The model under review builds one solid part; all positions refer to its coordinate system, in mm. Coordinates: 2 decimals unless noted, no trailing zeros. Write each loop counter-clockwise with the first axis right and the second up, starting at its lowest first coordinate (ties: lowest second). Pieces come first, ordered by that corner, then holes. Notation, with made-up numbers: (24.5, 41.5) - (79.5, 41.5) arc R26 ccw to (79.5, 63.5) - close; hole circle Ø1 at (76, -34.5). An arc over 180 degrees is marked (long way). Put each result on its own line as item: value. Start each with the question number.
Item 1: Consider section B-B on x = 0. Give the boundary of the cut face in (y, z), then the cut area to 3 significant figures.
Item 2: For pin 1 (6.5 mm diameter, centred on x = 2, y = -2, fed in from +Z) (3 decimals); pin 2 (6.5 mm diameter, centred on x = 0.5, y = -2.5, fed in from -Z) (3 decimals); pin 3 (4 mm diameter, centred on y = -6.5, z = -18, fed in from -X); pin 4 (6 mm diameter, centred on x = 2, z = -20.5, fed in from +Y), all flat-tipped, find the tip position at first contact; note any pin that passes through.
Item 3: To check wall thickness, follow L1, parallel to X at y = -5.75, z = 17 (3 decimals); L2, parallel to Z at x = -13, y = -4; L3, parallel to Z at x = -2.5, y = -2.25. State the ranges of each line that lie inside material, in increasing order. Write a range as [from, to].
Item 4: Consider section C-C on y = -3.5. State how many separate pieces and enclosed holes the cut face has, then the cut area to 3 significant figures.
Item 5: Consider section A-A on y = -8.25. Give the boundary of the cut face in (x, z) (1 decimal), then the cut area to 3 significant figures.
```python
from build123d import *

# Parameters (mm, degrees)
F0_R     = 29.845
F1_DEPTH = 6.35
F2_R     = 8.636
F3_DEPTH = 8.89
F4_R     = 1.5875
F5_DEPTH = 15.241
F6_R     = 1.4605
F7_DEPTH = 15.241
F8_R     = 1.4605
F9_DEPTH = 29.846


with BuildPart() as f1:
    # F0 (on Front) → F1 (new body)
    with BuildSketch(Plane.XZ):
        with Locations((0.718291, 0)):
            Circle(F0_R)
        Polygon((-12.740865, -24.658204), (-17.411727, -21.264625), (-16.808232, -15.52275), (-11.533875, -13.174455), (-6.863013, -16.568034), (-7.466508, -22.309909), align=None, mode=Mode.SUBTRACT)
        Polygon((-24.664124, -12.037813), (-26.448234, -6.546885), (-22.585007, -2.256337), (-16.937669, -3.456715), (-15.153559, -8.947643), (-19.016786, -13.238191), align=None, mode=Mode.SUBTRACT)
        Polygon((4.323334, -27.86), (-1.450169, -27.86), (-4.33692, -22.86), (-1.450169, -17.86), (4.323334, -17.86), (7.210085, -22.86), align=None, mode=Mode.SUBTRACT)
        Polygon((20.010529, -20.420223), (15.339667, -23.813802), (10.06531, -21.465507), (9.461815, -15.723632), (14.132676, -12.330053), (19.407034, -14.678348), align=None, mode=Mode.SUBTRACT)
        Polygon((28.328745, -5.180614), (26.544635, -10.671542), (20.897297, -11.87192), (17.034069, -7.581372), (18.81818, -2.090444), (24.465518, -0.890066), align=None, mode=Mode.SUBTRACT)
        Polygon((-26.892163, 5.180614), (-25.108052, 10.671542), (-19.460715, 11.87192), (-15.597487, 7.581372), (-17.381598, 2.090444), (-23.028935, 0.890066), align=None, mode=Mode.SUBTRACT)
        Polygon((-18.573947, 20.420223), (-13.903085, 23.813802), (-8.628728, 21.465507), (-8.025232, 15.723632), (-12.696094, 12.330053), (-17.970451, 14.678348), align=None, mode=Mode.SUBTRACT)
        Polygon((5.773503, 22.86), (2.886751, 17.86), (-2.886751, 17.86), (-5.773503, 22.86), (-2.886751, 27.86), (2.886751, 27.86), align=None, mode=Mode.SUBTRACT)
        Polygon((26.100706, 12.037813), (27.884817, 6.546885), (24.021589, 2.256337), (18.374252, 3.456715), (16.590141, 8.947643), (20.453368, 13.238191), align=None, mode=Mode.SUBTRACT)
        Polygon((14.177448, 24.658204), (18.848309, 21.264625), (18.244814, 15.52275), (12.970457, 13.174455), (8.299595, 16.568034), (8.90309, 22.309909), align=None, mode=Mode.SUBTRACT)
    extrude(amount=F1_DEPTH)

    # F2 (on face) → F3 (join)
    with BuildSketch(Plane.XZ.offset(6.35)):
        with Locations((0.718291, 0)):
            Circle(F2_R)
    extrude(amount=F3_DEPTH)

    # F4 (on face) → F5 (cut, through all)
    with BuildSketch(Plane.XZ.offset(15.24)):
        with Locations((0.718291, 0)):
            Circle(F4_R)
    extrude(amount=-F5_DEPTH, mode=Mode.SUBTRACT)

    # F6 (on face) → F7 (cut, through all)
    with BuildSketch(Plane(origin=(0, 0, 0), x_dir=(-1, 0, 0), z_dir=(0, 1, 0))):
        with Locations((9.9703, 0)):
            Circle(F6_R)
    extrude(amount=-F7_DEPTH, mode=Mode.SUBTRACT)

    # F8 (on Top) → F9 (cut, through all)
    with BuildSketch(Plane.XY):
        with Locations((0, -11.241886)):
            Circle(F8_R)
    extrude(amount=F9_DEPTH, mode=Mode.SUBTRACT)


solid = f1.part
```
Report:
1. outline: (-15.24, -8.61) - (-6.35, -8.61) - (-6.35, -17.86) - (0, -17.86) - (0, -1.42) - (-15.24, -1.42) - close; (-15.24, 1.42) - (-12.7, 1.42) - (-12.7, 8.61) - (-15.24, 8.61) - close; (-9.78, 1.42) - (0, 1.42) - (0, 17.86) - (-6.35, 17.86) - (-6.35, 8.61) - (-9.78, 8.61) - close; (-6.35, -29.84) - (0, -29.84) - (0, -27.86) - (-6.35, -27.86) - close; (-6.35, 27.86) - (0, 27.86) - (0, 29.84) - (-6.35, 29.84) - close
1. area: 341 mm²
2. pin 1: z = 29.845
2. pin 2: z = -29.845
2. pin 3: x = -24.47
2. pin 4: y = 0
3. L1: [-23.812, -18.214], [-8.159, 8.345], [18.4, 25.248]
3. L2: [-26.51, -24.47], [-13.83, 12.47], [23.41, 26.51]
3. L3: [-29.67, -26.04], [-19.68, 17.86], [27.86, 29.67]
4. separate pieces: 1
4. enclosed holes: 12
4. area: 1,920 mm²
5. outline: circle Ø17.3 at (0.7, 0); hole circle Ø3.2 at (0.7, 0)
5. area: 226 mm²
